Build history of the part. All positions in model axes, mm. Coordinates: 2 decimals unless noted, no trailing zeros. Write each loop counter-clockwise with the first axis right and the second up, starting at its lowest first coordinate (ties: lowest second). Pieces come first, ordered by that corner, then holes. Notation, with made-up numbers: (71, 74.25) -> (95, 74.25) arc R12 cw to (95, 91.25) -> close; hole circle Ø10 at (-20.5, -23). An arc over 180 degrees is marked (long way). Write each question's results on one line, items separated by ' | '. Start each with the question number.
Q1. Saw through at B-B on z = -10. Give the cut face in (x, y).
Q2. Drop flat-ended pins along their axis: pin 1 Ø1 at (x, y) = (22, 1.5) entering from -Z; pin 2 Ø5 at (x, z) = (0, -58) entering from -Y; pin 3 Ø1 at (x, y) = (20, 1.5) entering from +Z; pin 4 Ø12 at (x, z) = (23, 6.5) entering from +Y. Give the stop position or say it passes through.
Q3. Saw through at C-C on y = 0.45. Give the cut face in (x, z).
Q4. Drill centre lines: line 1 (X direction, y = 1.7, z = -10); line 2 (X direction, y = 1.55, z = 58); line 3 (Z direction, x = 0, y = 1.5). Where is each one in solid material? Low to high.
Q5. Saw through at A-A on x = 25. Give the cut face in (y, z).
Q6. Saw through at D-D on z = 58. Give the cut face in (x, y), and give its area (3 significant figures).
Q7. Two-plate mould, pull along X, no slides. Class faces 1 (the face through (0, 2, -1)), 2 (the face through (0.45, 1.65, 59.43)): released by +X, released by -X, zero draft, split by the parting line, or undercut.
from build123d import *

# Parameters (mm, degrees)
SKETCH1_R                     = 1.5
BOSS_EXTRUDE1_DEPTH           = 2
CSK_FOR_M3_SFHCS1_D           = 3
CSK_FOR_M3_SFHCS1_DEPTH       = 9.5
CSK_FOR_M3_SFHCS1_CSINK_D     = 5.6
CSK_FOR_M3_SFHCS1_CSINK_ANGLE = 90
CSK_FOR_M3_SFHCS1_TIP         = 0.901290929


with BuildPart() as part:
    # Sketch1 → Boss-Extrude1 (new body)
    with BuildSketch(Plane(origin=(0, 0, 0), x_dir=(1, 0, 0), z_dir=(0, 1, 0))):
        with BuildLine():
            Line((12, 17.5), (27, 17.5))
            ThreePointArc((27, 17.5), (28.414213562, 16.914213562), (29, 15.5))
            Line((29, 15.5), (29, 4.5))
            ThreePointArc((29, 4.5), (28.414213562, 3.085786438), (27, 2.5))
            Line((27, 2.5), (12, 2.5))
            ThreePointArc((12, 2.5), (10.585786438, 1.914213562), (10, 0.5))
            Line((10, 0.5), (10, -60))
            ThreePointArc((10, -60), (9.414213562, -61.414213562), (8, -62))
            Line((8, -62), (-8, -62))
            ThreePointArc((-8, -62), (-9.414213562, -61.414213562), (-10, -60))
            Line((-10, -60), (-10, 0.5))
            ThreePointArc((-10, 0.5), (-10.585786438, 1.914213562), (-12, 2.5))
            Line((-12, 2.5), (-27, 2.5))
            ThreePointArc((-27, 2.5), (-28.414213562, 3.085786438), (-29, 4.5))
            Line((-29, 4.5), (-29, 15.5))
            ThreePointArc((-29, 15.5), (-28.414213562, 16.914213562), (-27, 17.5))
            Line((-27, 17.5), (-12, 17.5))
            ThreePointArc((-12, 17.5), (-10.585786438, 18.085786438), (-10, 19.5))
            Line((-10, 19.5), (-10, 60))
            ThreePointArc((-10, 60), (-9.414213562, 61.414213562), (-8, 62))
            Line((-8, 62), (8, 62))
            ThreePointArc((8, 62), (9.414213562, 61.414213562), (10, 60))
            Line((10, 60), (10, 19.5))
            ThreePointArc((10, 19.5), (10.585786438, 18.085786438), (12, 17.5))
        make_face()
        with Locations(Location((0, 58, 0), (0, 0, 270))):
            Circle(SKETCH1_R, mode=Mode.SUBTRACT)
        with Locations(Location((0, -58, 0), (0, 0, 270))):
            Circle(SKETCH1_R, mode=Mode.SUBTRACT)
        with Locations(Location((25, 10, 0), (0, 0, 270))):
            Circle(SKETCH1_R, mode=Mode.SUBTRACT)
        with Locations(Location((-25, 10, 0), (0, 0, 270))):
            Circle(SKETCH1_R, mode=Mode.SUBTRACT)
    extrude(amount=BOSS_EXTRUDE1_DEPTH)

    # CSK for M3 SFHCS1
    with Locations(Plane(origin=(25, 0, -10), x_dir=(0, 0, -1), z_dir=(0, -1, 0))):
        with Locations((0, 0), (0, -50), (-68, -25), (48, -25)):
            CounterSinkHole(CSK_FOR_M3_SFHCS1_D / 2, CSK_FOR_M3_SFHCS1_CSINK_D / 2, depth=CSK_FOR_M3_SFHCS1_DEPTH, counter_sink_angle=CSK_FOR_M3_SFHCS1_CSINK_ANGLE)
            with Locations((0, 0, -(CSK_FOR_M3_SFHCS1_DEPTH + CSK_FOR_M3_SFHCS1_TIP / 2))):  # 118° drill point
                Cone(0, CSK_FOR_M3_SFHCS1_D / 2, CSK_FOR_M3_SFHCS1_TIP, mode=Mode.SUBTRACT)


solid = part.part
Returned:
1) outline: (-29, 0) -> (-27.8, 0) -> (-26.5, 1.3) -> (-26.5, 2) -> (-29, 2) -> close; (-23.5, 1.3) -> (-22.2, 0) -> (22.2, 0) -> (23.5, 1.3) -> (23.5, 2) -> (-23.5, 2) -> close; (26.5, 1.3) -> (27.8, 0) -> (29, 0) -> (29, 2) -> (26.5, 2) -> close
2) pin 1: stops at z = -17.5 | pin 2: stops at y = 0.3 | pin 3: stops at z = -2.5 | pin 4: passes through
3) outline: (-29, -15.5) arc R2 ccw to (-27, -17.5) -> (-12, -17.5) arc R2 cw to (-10, -19.5) -> (-10, -60) arc R2 ccw to (-8, -62) -> (8, -62) arc R2 ccw to (10, -60) -> (10, -19.5) arc R2 cw to (12, -17.5) -> (27, -17.5) arc R2 ccw to (29, -15.5) -> (29, -4.5) arc R2 ccw to (27, -2.5) -> (12, -2.5) arc R2 cw to (10, -0.5) -> (10, 60) arc R2 ccw to (8, 62) -> (-8, 62) arc R2 ccw to (-10, 60) -> (-10, -0.5) arc R2 cw to (-12, -2.5) -> (-27, -2.5) arc R2 ccw to (-29, -4.5) -> close; hole circle Ø4.7 at (-25, -10); hole circle Ø4.7 at (0, -58); hole circle Ø4.7 at (0, 58); hole circle Ø4.7 at (25, -10)
4) line 1: x = -29 to -26.5, -23.5 to 23.5, 26.5 to 29 | line 2: x = -10 to -1.5, 1.5 to 10 | line 3: z = -62 to -59.5, -56.5 to 56.5, 59.5 to 62
5) outline: (0, -17.5) -> (2, -17.5) -> (2, -11.5) -> (1.3, -11.5) -> (0, -12.8) -> close; (0, -7.2) -> (1.3, -8.5) -> (2, -8.5) -> (2, -2.5) -> (0, -2.5) -> close
6) outline: (-10, 0) -> (-2.8, 0) -> (-1.5, 1.3) -> (-1.5, 2) -> (-10, 2) -> close; (1.5, 1.3) -> (2.8, 0) -> (10, 0) -> (10, 2) -> (1.5, 2) -> close | area: 32.3 mm2
7) face 1: zero draft | face 2: undercut
